Input: dimensioned drawing with shaded views. Units: mm. Origin: part minimum x, y, z. A direction names the side the tool comes from. Round coordinates to 2 decimals unless told otherwise and drop trailing zeros. Loops run counter-clockwise (first coordinate to the right, second up) from the corner with the lowest first, then second, coordinate; pieces in that order, holes last. Notation, with made-up numbers: (10.5, 21.25) - (26.5, 21.25) arc R22 cw to (26.5, 58.25) - close; hole circle Ø1 at (51.25, 42). An arc over 180 degrees is marked (long way). Use CSV: the item, a comma, the result in double quotes. Start each with the question number.
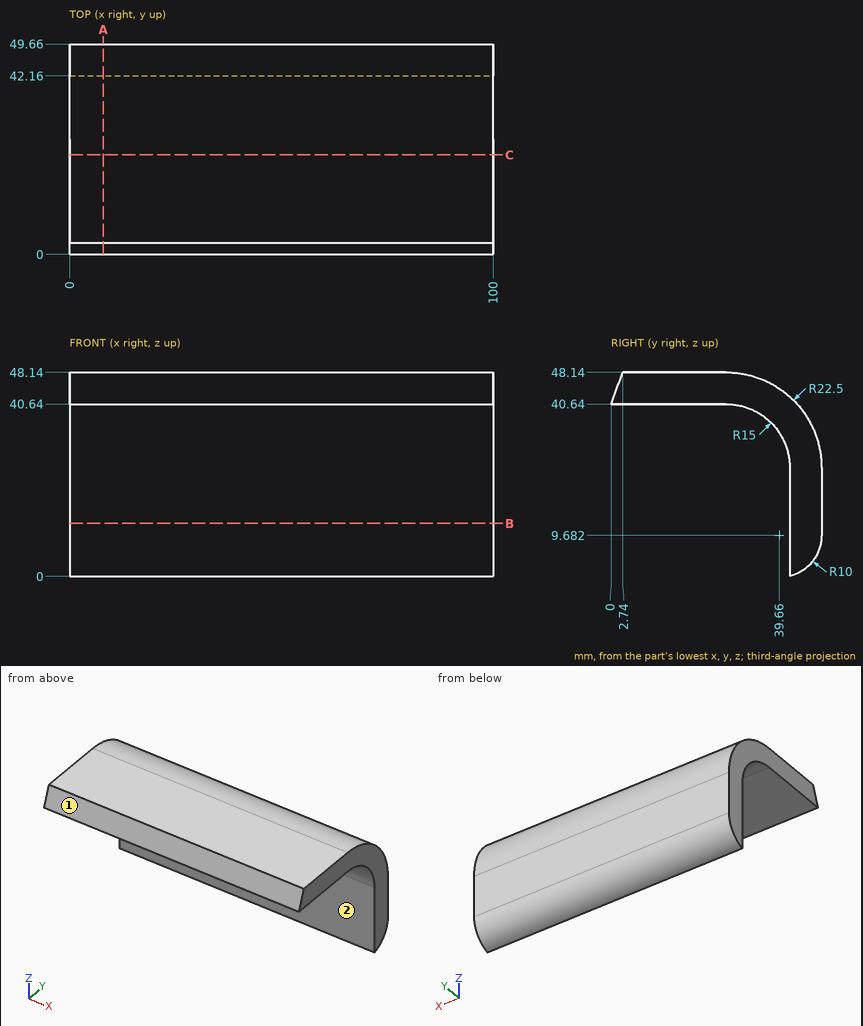
1. Contact query for flat-ended pins moving along their axis: P1, Ø2, axis at x = 64.5, z = 29.5, coming from the -Y side; P2, Ø8, axis at x = 27.5, y = 20, coming from the -Z side; P3, Ø20.5, axis at x = 74.5, z = 11, coming from the -Y side. Output: stop coordinate, or through.
2. Section query A-A on x = 8. Return the cut outline in (y, z), and give its area (3 significant figures).
3. Line query: line 1 along Z through (x, y) = (62.5, 11); line 2 along Y through (x, z) = (65, 12.5); line 3 along Y through (x, z) = (46.5, 41). Output: solid intervals per line, ascending.
4. Section query B-B on z = 12.5. Return the cut outline in (x, y), and give its area (3 significant figures).
5. Section query C-C on y = 23.5. Return the cut outline in (x, z).
6. Reachability of the marked faces 1 and 2 from +Z, -Z, +X, -X, +Y, -Y: full face, straight path, thin tool, end or side. Return the list, or none.
Values:
1,P1,"stops at y = 41.35"
1,P2,"stops at z = 40.64"
1,P3,"stops at y = 42.16"
2,outline,"(0, 40.64) - (27.16, 40.64) arc R15 cw to (42.16, 25.64) - (42.16, 0) arc R10 ccw to (49.66, 9.68) - (49.66, 25.64) arc R22.5 ccw to (27.16, 48.14) - (2.74, 48.14) - close"
2,area,"588 mm^2"
3,line 1,"z = 40.64 to 48.14"
3,line 2,"y = 42.16 to 49.66"
3,line 3,"y = 0.13 to 43.6"
4,outline,"(0, 42.16) - (100, 42.16) - (100, 49.66) - (0, 49.66) - close"
4,area,"750 mm^2"
5,outline,"(0, 40.64) - (100, 40.64) - (100, 48.14) - (0, 48.14) - close"
6,face 1,"+Z, +X, -X, -Y"
6,face 2,"-Z, +X, -X, -Y"
